The listing builds one solid part. Answer for the finished solid, in the listing's coordinates (mm). Face numbers are marked on the shaded views. A direction names the side the tool comes from. Give positions to 0.01 mm unless a question says otherwise; leave off trailing zeros. Loops run counter-clockwise (first coordinate to the right, second up) from the corner with the lowest first, then second, coordinate; pieces in that order, holes last.
Item 1: Consider line 1 along X through (y, z) = (17, 13); line 2 along X through (y, z) = (29.5, 8.5) (3 decimals); line 3 along Y through (x, z) = (-17.5, 16.5). Determine where each line is inside the solid, lowest interval first.
Item 2: The mould has two halves that part along X. Classify the marked faces 1, 2, 3 and 4: pulls with the +X half, pulls with the -X half, needs draft (parallel to the pull), parting line crosses it, or undercut.
Item 3: Each of these flat-tipped pins is pushed along its axis until it touches: pin 1 Ø6 at (x, y) = (4.5, 16.5) entering from +Z; pin 2 Ø2 at (y, z) = (15.5, 13.5) entering from -X; pin 3 Ø6.5 at (x, y) = (-8.5, 16.5) entering from +Z. Where does it stop, or does it pass through?
Item 4: Section A-A, the plane z = 8 is taken. Give the vertices of the cut face in (x, y) (3 decimals).
Item 5: Section C-C, the plane z = 15 is taken. Give the vertices of the cut face in (x, y).
Item 6: A tool of negligible diameter and unlimited length cuts with its end or side. For the marked faces 5 and 6, from which of +Z, -Z, +X, -X, +Y, -Y can it reach the whole face along a straight path? Write none if from no direction.
Item 7: Section D-D, the plane z = -1 is taken. Give the vertices of the cut face in (x, y) (1 decimal).
from build123d import *

# Parameters (mm, degrees)
BOSS_EXTRUDE1_DEPTH                            = 31.75
CBORE_FOR_8_SOCKET_HEAD_CAP_SCREW1_D           = 4.9149
CBORE_FOR_8_SOCKET_HEAD_CAP_SCREW1_CBORE_D     = 7.9375
CBORE_FOR_8_SOCKET_HEAD_CAP_SCREW1_CBORE_DEPTH = 4.1656
CUT_EXTRUDE1_DEPTH                             = 32.7500001
CUT_EXTRUDE3_DEPTH                             = 77.2000001
FILLET1_R                                      = 2.54
FILLET2_R                                      = 2.54
FILLET3_R                                      = 2.54


with BuildPart() as part:
    # Sketch1 → Boss-Extrude1 (new body)
    with BuildSketch(Plane(origin=(0, 0, 0), x_dir=(1, 0, 0), z_dir=(0, 1, 0))):
        with BuildLine():
            Line((38.1, 15.875), (38.1, -19.05))
            Line((38.1, -19.05), (12.7, -19.05))
            Line((12.7, -19.05), (12.7, -9.525))
            Line((12.7, -9.525), (22.225, -9.525))
            Line((22.225, -9.525), (22.225, 0))
            Line((22.225, 0), (-22.225, 0))
            Line((-22.225, 0), (-22.225, -9.525))
            Line((-22.225, -9.525), (-12.7, -9.525))
            Line((-12.7, -9.525), (-12.7, -19.05))
            Line((-12.7, -19.05), (-38.1, -19.05))
            Line((-38.1, -19.05), (-38.1, 15.875))
            ThreePointArc((-38.1, 15.875), (0, 11.035665491), (38.1, 15.875))
        make_face()
    extrude(amount=BOSS_EXTRUDE1_DEPTH)

    # CBORE for #8 Socket Head Cap Screw1 (through all)
    with Locations(Plane.XY):
        with Locations((-8.5725, 15.875), (8.5725, 15.875)):
            CounterBoreHole(CBORE_FOR_8_SOCKET_HEAD_CAP_SCREW1_D / 2, CBORE_FOR_8_SOCKET_HEAD_CAP_SCREW1_CBORE_D / 2, CBORE_FOR_8_SOCKET_HEAD_CAP_SCREW1_CBORE_DEPTH)

    # Sketch4 → Cut-Extrude1 (cut, through all)
    with BuildSketch(Plane(origin=(0, 31.75, 0), x_dir=(1, 0, 0), z_dir=(0, 1, 0))):
        with BuildLine():
            Line((-38.1, -19.05), (-38.1, 3.649511931))
            ThreePointArc((-38.1, 3.649511931), (-31.500580819, -8.639700689), (-22.216037286, -19.05))
            Line((-22.216037286, -19.05), (-38.1, -19.05))
        make_face()
    cut_extrude1 = extrude(amount=-CUT_EXTRUDE1_DEPTH, mode=Mode.SUBTRACT)

    # Mirror1: Cut-Extrude1 across plane
    add(cut_extrude1.mirror(Plane(origin=(0, 0, 0), x_dir=(0, 0, 1), z_dir=(1, 0, 0))), mode=Mode.SUBTRACT)

    # Sketch5 → Cut-Extrude3 (cut, through all)
    with BuildSketch(Plane.ZY.offset(38.1)):
        with BuildLine():
            Line((-3.649511931, 31.75), (19.05, 31.75))
            Line((19.05, 31.75), (19.05, 24.4475))
            ThreePointArc((19.05, 24.4475), (8.273096301, 29.879437004), (-3.649511931, 31.75))
        make_face()
        with BuildLine():
            ThreePointArc((19.05, 7.3025), (8.273096301, 1.870562996), (-3.649511931, 0))
            Line((-3.649511931, 0), (19.05, 0))
            Line((19.05, 0), (19.05, 7.3025))
        make_face()
    extrude(amount=-CUT_EXTRUDE3_DEPTH, mode=Mode.SUBTRACT)

    # Fillet1
    fillet1_edges = [part.edges().sort_by_distance(p)[0] for p in [
        (0, 0, -11.035665491),
        (38.1, 15.875, -15.875),
        (-38.1, 15.875, -15.875),
        (0, 31.75, -11.035665491),
    ]]
    fillet(fillet1_edges, radius=FILLET1_R)

    # Fillet2
    fillet2_edges = [part.edges().sort_by_distance(p)[0] for p in [
        (12.7, 15.875, 19.05),
        (12.7, 15.875, 9.525),
        (-12.7, 15.875, 9.525),
        (-12.7, 15.875, 19.05),
    ]]
    fillet(fillet2_edges, radius=FILLET2_R)

    # Fillet3
    fillet3_edges = [part.edges().sort_by_distance(p)[0] for p in [
        (22.216037286, 15.875, 19.05),
        (-22.216037286, 15.875, 19.05),
    ]]
    fillet(fillet3_edges, radius=FILLET3_R)


solid = part.part
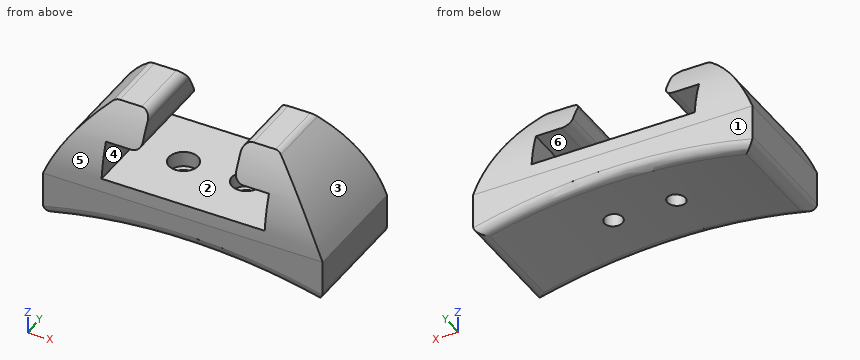
Worked answers:
1. line 1: x = -28.14 to -12.7, 12.7 to 28.14
1. line 2: x = -31.598 to -22.225, 22.225 to 31.598
1. line 3: y = 5.62 to 26.13
2. face 1: needs draft
2. face 2: undercut
2. face 3: pulls with the +X half
2. face 4: undercut
3. pin 1: stops at z = 0
3. pin 2: stops at x = -28.56
3. pin 3: stops at z = -4.17
4. outline: (-31.942, 1.784) - (-22.225, 1.784) - (-22.225, 29.966) - (-31.942, 29.966) - close; (22.225, 1.784) - (31.942, 1.784) - (31.942, 29.966) - (22.225, 29.966) - close
5. outline: (-26.36, 4.76) - (-12.7, 4.76) - (-12.7, 26.99) - (-26.36, 26.99) - close; (12.7, 4.76) - (26.36, 4.76) - (26.36, 26.99) - (12.7, 26.99) - close
6. face 5: +Z, +X, -X, -Y
6. face 6: +Y, -Y
7. outline: (-37, 0.1) - (37, 0.1) - (37, 31.7) - (-37, 31.7) - close; hole circle Ø7.9 at (-8.6, 15.9); hole circle Ø7.9 at (8.6, 15.9)
